Model file for the job. Use its own axes, mm. A direction names the side the tool comes from. Give positions to 0.01 mm unless a question says otherwise; leave off trailing zeros. Write each loop counter-clockwise with the first axis right and the second up, starting at its lowest first coordinate (ties: lowest second). Pieces come first, ordered by that corner, then holes.
```python
from build123d import *

# Parameters (mm, degrees)
F0_W     = 138.5
F0_H     = 69.5
F1_DEPTH = 40
F2_W     = 133.5
F2_H     = 64.5
F3_DEPTH = 37.5
F4_W     = 132
F4_H     = 62.5
F5_DEPTH = 2.5
F6_W     = 8
F6_H     = 8
F7_DEPTH = 138.5
F8_W     = 8
F8_H     = 8
F9_DEPTH = 69.5


with BuildPart() as f1:
    # F0 (on Top) → F1 (new body)
    with BuildSketch(Plane.XY):
        with Locations((69.25, 34.75)):
            Rectangle(F0_W, F0_H)
    extrude(amount=F1_DEPTH)

    # F2 (on face) → F3 (cut)
    with BuildSketch(Plane.XY.offset(40)):
        with Locations((69.25, 34.75)):
            Rectangle(F2_W, F2_H)
    extrude(amount=-F3_DEPTH, mode=Mode.SUBTRACT)

    # F4 (on face) → F5 (join)
    with BuildSketch(Plane(origin=(0, 0, 0), x_dir=(1, 0, 0), z_dir=(0, 0, -1))):
        with Locations((69.25, -34.75)):
            Rectangle(F4_W, F4_H)
    extrude(amount=F5_DEPTH)

    # F6 (on face) → F7 (cut)
    with BuildSketch(Plane.YZ.offset(138.5)):
        with Locations((11.25, 30)):
            Rectangle(F6_W, F6_H)
        with Locations((11.25, 10)):
            Rectangle(F6_W, F6_H)
        with Locations((57.25, 10)):
            Rectangle(F6_W, F6_H)
        with Locations((57.25, 30)):
            Rectangle(F6_W, F6_H)
        with Locations((34.25, 30)):
            Rectangle(F6_W, F6_H)
        with Locations((34.25, 10)):
            Rectangle(F6_W, F6_H)
    extrude(amount=-F7_DEPTH, mode=Mode.SUBTRACT)

    # F8 (on face) → F9 (cut)
    with BuildSketch(Plane.XZ):
        with Locations((10, 30)):
            Rectangle(F8_W, F8_H)
        with Locations((10, 10)):
            Rectangle(F8_W, F8_H)
        with Locations((29.75, 10)):
            Rectangle(F8_W, F8_H)
        with Locations((29.75, 30)):
            Rectangle(F8_W, F8_H)
        with Locations((49.5, 30)):
            Rectangle(F8_W, F8_H)
        with Locations((49.5, 10)):
            Rectangle(F8_W, F8_H)
        with Locations((69.25, 10)):
            Rectangle(F8_W, F8_H)
        with Locations((69.25, 30)):
            Rectangle(F8_W, F8_H)
        with Locations((89, 30)):
            Rectangle(F8_W, F8_H)
        with Locations((89, 10)):
            Rectangle(F8_W, F8_H)
        with Locations((108.75, 10)):
            Rectangle(F8_W, F8_H)
        with Locations((108.75, 30)):
            Rectangle(F8_W, F8_H)
        with Locations((128.5, 30)):
            Rectangle(F8_W, F8_H)
        with Locations((128.5, 10)):
            Rectangle(F8_W, F8_H)
    extrude(amount=-F9_DEPTH, mode=Mode.SUBTRACT)


solid = f1.part
```
1. Slice it at C-C, the plane z = 4. Write the cut outline in (x, y).
Calculated:
outline: (0, 0) - (138.5, 0) - (138.5, 69.5) - (0, 69.5) - close; hole (2.5, 2.5) - (136, 2.5) - (136, 67) - (2.5, 67) - close
2. Pin check, flat tips, straight feed: P1, Ø1.2, axis at y = 67.5, z = 29, coming from the -X side; P2, Ø4, axis at x = 21, y = 29, coming from the +Z side; P3, Ø1.2, axis at x = 1.5, y = 59, coming from the -Z side. Stop position of each tip, or through.
Calculated:
P1: stops at x = 0
P2: stops at z = 2.5
P3: stops at z = 0
3. Which spindle directions (+Z, -Z, +X, -X, +Y, -Y) get a long thin tool onto all of the face, cutting with end or side? Do faces 3 (the flat face through (1, 7.25, 30)), 4 (the flat face through (69, 1, 6)), 5 (the flat face through (68, 34, -2.5)). Say none if no direction does.
Calculated:
face 3: +X, -X
face 4: +Y, -Y
face 5: -Z, +X, -X, +Y, -Y
4. Slice it at B-B, the plane y = 13.5. Write the cut outline in (x, z), and give its area (3 significant figures).
Calculated:
outline: (0, 0) - (3.25, 0) - (3.25, -2.5) - (135.25, -2.5) - (135.25, 0) - (138.5, 0) - (138.5, 6) - (136, 6) - (136, 2.5) - (2.5, 2.5) - (2.5, 6) - (0, 6) - close; (0, 14) - (2.5, 14) - (2.5, 26) - (0, 26) - close; (0, 34) - (2.5, 34) - (2.5, 40) - (0, 40) - close; (136, 14) - (138.5, 14) - (138.5, 26) - (136, 26) - close; (136, 34) - (138.5, 34) - (138.5, 40) - (136, 40) - close
area: 784 mm2
5. Slice it at D-D, the plane x = 20. Write the cut outline in (y, z).
Calculated:
outline: (0, 0) - (3.5, 0) - (3.5, -2.5) - (66, -2.5) - (66, 0) - (69.5, 0) - (69.5, 40) - (67, 40) - (67, 2.5) - (2.5, 2.5) - (2.5, 40) - (0, 40) - close
6. Slice it at A-A, the plane x = 111. Write the cut outline in (y, z), and give its area (4 significant figures).
Calculated:
outline: (0, 0) - (3.5, 0) - (3.5, -2.5) - (66, -2.5) - (66, 0) - (69.5, 0) - (69.5, 6) - (67, 6) - (67, 2.5) - (2.5, 2.5) - (2.5, 6) - (0, 6) - close; (0, 14) - (2.5, 14) - (2.5, 26) - (0, 26) - close; (0, 34) - (2.5, 34) - (2.5, 40) - (0, 40) - close; (67, 14) - (69.5, 14) - (69.5, 26) - (67, 26) - close; (67, 34) - (69.5, 34) - (69.5, 40) - (67, 40) - close
area: 437.5 mm2
7. Pull direction X, two halves, no side cores. Call faces 1 (the flat face through (30, 68, 6)), 2 (the flat face through (1, 7.25, 10)): +X half, -X half, draft (parallel to the pull), parting line (faces both ways), or undercut.
Calculated:
face 1: undercut
face 2: draft
8. Probe probe 1 along Y at (x, z) = (94.5, 9.5); probe 2 along X at (y, z) = (23.5, 32); probe 3 along Z at (x, y) = (36, 16). List the from-to ranges inside material, lowest first.
Calculated:
probe 1: y = 0 to 2.5, 67 to 69.5
probe 2: x = 0 to 2.5, 136 to 138.5
probe 3: z = -2.5 to 2.5
